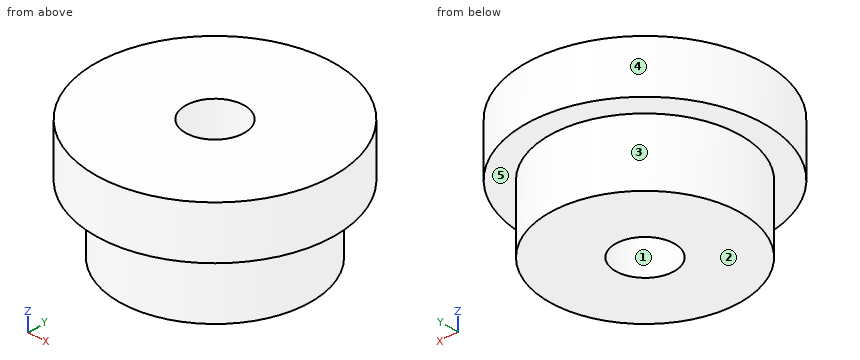
Autodesk Inventor part; units mm, degrees
ref_plane "YZ Plane" through (0, 0, 0) normal (1, 0, 0) x (0, 1, 0)
ref_plane "XZ Plane" through (0, 0, 0) normal (0, 1, 0) x (-1, 0, 0)
ref_plane "XY Plane" through (0, 0, 0) normal (0, 0, 1) x (1, 0, 0)
sketch "スケッチ1" plane through (0, 0, 0) normal (0, 0, 1) x (1, 0, 0)
  circle A0 centre (0, 0) radius 5
  dimension "d0" = 10
extrude "押し出し1" add sketch "スケッチ1" along normal blind 2.2
sketch "スケッチ2" plane through (0, 0, 0) normal (0, 0, -1) x (-1, 0, 0)
  circle A0 centre (0, 0) radius 4
  dimension "d3" = 8
extrude "押し出し2" add sketch "スケッチ2" along normal blind 2.8
sketch "スケッチ3" plane through (0, 0, -2.8) normal (0, 0, -1) x (-1, 0, 0)
  point P0 (0, 0)
  point P1 (0, 0)
hole "穴1" at (0, 0, -2.8) direction (0, 0, 1) diameter 2.459 end through all
properties part number "link2part7" material "アルミニウム 6061"
For this review, take the finished solid that the model builds, in its own axes (mm). Face numbers are marked on the shaded views. A direction names the side the tool comes from. Round coordinates to 2 decimals unless told otherwise and drop trailing zeros. Loops run counter-clockwise (first coordinate to the right, second up) from the corner with the lowest first, then second, coordinate; pieces in that order, holes last.
Q1. Mouldability with a two-part tool opening along Y and no side actions: class the marked faces 1, 2 and 3 as +Y half, -Y half, draft (parallel to the pull), parting line (faces both ways), or undercut.
Result sheet:
face 1: undercut
face 2: draft
face 3: parting line
Q2. Machinability: for the marked faces 4 and 5, which of the approach directions +Z, -Z, +X, -X, +Y, -Y give a long, thin tool a straight path to every point of the face, cutting with its end or side? Answer none if there is none.
Result sheet:
face 4: +Z, -Z
face 5: -Z
Q3. Add section A-A on y = 0. Write out the cut boundary in (x, z).
Result sheet:
outline: (-5, 0) - (-4, 0) - (-4, -2.8) - (-1.23, -2.8) - (-1.23, 2.2) - (-5, 2.2) - close; (1.23, -2.8) - (4, -2.8) - (4, 0) - (5, 0) - (5, 2.2) - (1.23, 2.2) - close
Q4. Add section D-D on x = -3.25. Write out the cut boundary in (y, z).
Result sheet:
outline: (-3.8, 0) - (-2.33, 0) - (-2.33, -2.8) - (2.33, -2.8) - (2.33, 0) - (3.8, 0) - (3.8, 2.2) - (-3.8, 2.2) - close
Q5. To check wall thickness, follow line 1 along Y through (x, z) = (0, 0.3); line 2 along Y through (x, z) = (0, -0.6); line 3 along X through (y, z) = (-0.75, -1.7). State the ranges of each line that lie inside material, in increasing order.
Result sheet:
line 1: y = -5 to -1.23, 1.23 to 5
line 2: y = -4 to -1.23, 1.23 to 4
line 3: x = -3.93 to -0.97, 0.97 to 3.93
Q6. Add section C-C on z = 1.95. Write out the cut boundary in (x, y), plus the area to 3 significant figures.
Result sheet:
outline: circle Ø10 at (0, 0); hole circle Ø2.46 at (0, 0)
area: 73.8 mm2
Q7. Insertion check: pin 1 Ø1.5 at (x, y) = (0, 0) entering from -Z; pin 2 Ø1.5 at (x, y) = (4, 3.5) entering from +Z; pin 3 Ø1 at (y, z) = (2.5, -1) entering from +X; pin 4 Ø2 at (x, z) = (-3, 0.5) entering from -Y. Each pin has a flat end and moves straight along its axis. Give the tip position at first contact, or say it passes through.
Result sheet:
pin 1: passes through
pin 2: stops at z = 2.2
pin 3: stops at x = 3.46
pin 4: stops at y = -4.58
